Model file for the job. Use its own axes, mm. Face numbers are marked on the shaded views. A direction names the side the tool comes from. Give positions to 0.01 mm unless a question says otherwise; leave off trailing zeros. Loops run counter-clockwise (first coordinate to the right, second up) from the corner with the lowest first, then second, coordinate; pieces in that order, holes last. Notation, with made-up numbers: (-21.75, 14) - (7.25, 14) arc R20 cw to (7.25, 36) - close; hole circle Ø7 at (54.25, -21.75). An arc over 180 degrees is marked (long way). Use a Markdown table: item, result.
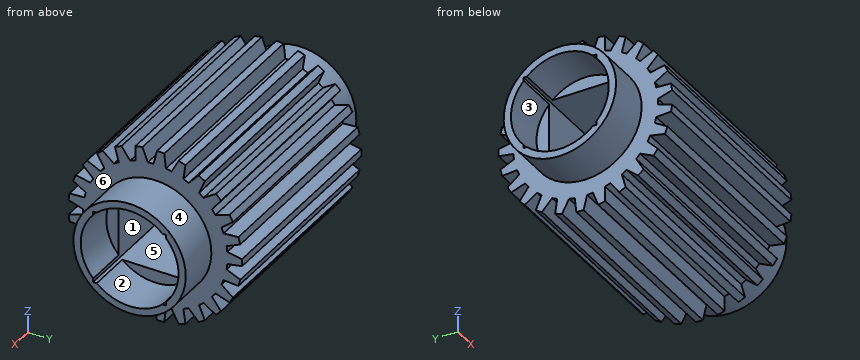
from build123d import *

# Parameters (mm, degrees)
BOSS_EXTRUDE2_START      = -9
BOSS_EXTRUDE2_DEPTH      = 14
BOSS_EXTRUDE3_DEPTH      = 5
BOSS_EXTRUDE3_DEPTH_BACK = 9
SKETCH3_R                = 5
CIRPATTERN1_COUNT        = 25
SKETCH4_W                = 5
SKETCH4_H                = 5
CUT_EXTRUDE1_DEPTH       = 18
BOSS_EXTRUDE4_DEPTH      = 3
BOSS_EXTRUDE4_DEPTH_BACK = 17
SKETCH6_R                = 3.881431072
SKETCH6_R_2              = 3.381431072
CUT_EXTRUDE2_DEPTH       = 10
CUT_EXTRUDE2_DEPTH_BACK  = 20
SKETCH7_W                = 5
SKETCH7_H                = 5.021637953


with BuildPart() as part:
    # Sketch2 → Boss-Extrude2 (new body)
    with BuildSketch(Plane(origin=(0, 0, 0), x_dir=(0, 0, -1), z_dir=(1, 0, 0)).offset(BOSS_EXTRUDE2_START)):
        with BuildLine():
            ThreePointArc((0.429587035, 4.981511315), (0, 5), (-0.429587035, 4.981511315))
            Line((-0.429587035, 4.981511315), (-0.700772987, 3.443539352))
            Line((-0.700772987, 3.443539352), (0.700772987, 3.443539352))
            Line((0.700772987, 3.443539352), (0.429587035, 4.981511315))
        make_face()
        with BuildLine():
            Line((0.25, 6), (-0.25, 6))
            Line((-0.25, 6), (-0.429587035, 4.981511315))
            ThreePointArc((-0.429587035, 4.981511315), (0, 5), (0.429587035, 4.981511315))
            Line((0.429587035, 4.981511315), (0.25, 6))
        make_face()
    boss_extrude2 = extrude(amount=BOSS_EXTRUDE2_DEPTH)

    # Sketch3 → Boss-Extrude3 (add, two sides: drawn at the far end of the back side and taken through both)
    with BuildSketch(Plane(origin=(0, 0, 0), x_dir=(0, 0, -1), z_dir=(1, 0, 0)).offset(-BOSS_EXTRUDE3_DEPTH_BACK)):
        Circle(SKETCH3_R)
    extrude(amount=BOSS_EXTRUDE3_DEPTH + BOSS_EXTRUDE3_DEPTH_BACK)

    # CirPattern1: Boss-Extrude2 ×25 about axis
    cirpattern1_axis = Axis((0, 0, 0), (1, 0, 0))
    for i in range(1, CIRPATTERN1_COUNT):
        add(boss_extrude2.rotate(cirpattern1_axis, i * 360 / CIRPATTERN1_COUNT))

    # Sketch4 → Cut-Extrude1 (cut)
    with BuildSketch(Plane(origin=(5, 0, 0), x_dir=(0, 0, -1), z_dir=(1, 0, 0))):
        Rectangle(SKETCH4_W, SKETCH4_H)
    extrude(amount=-CUT_EXTRUDE1_DEPTH, mode=Mode.SUBTRACT)

    # Sketch6 → Boss-Extrude4 (add, two sides: drawn at the far end of the back side and taken through both)
    with BuildSketch(Plane(origin=(5, 0, 0), x_dir=(0, 0, -1), z_dir=(1, 0, 0)).offset(-BOSS_EXTRUDE4_DEPTH_BACK)):
        Circle(SKETCH6_R)
        Circle(SKETCH6_R_2, mode=Mode.SUBTRACT)
    extrude(amount=BOSS_EXTRUDE4_DEPTH + BOSS_EXTRUDE4_DEPTH_BACK)

    # Sketch7 → Cut-Extrude2 (cut, two sides: drawn at the far end of the back side and taken through both)
    with BuildSketch(Plane(origin=(5, 0, 0), x_dir=(0, 0, -1), z_dir=(1, 0, 0)).offset(-CUT_EXTRUDE2_DEPTH_BACK)):
        with Locations((0, -0.010818977)):
            Rectangle(SKETCH7_W, SKETCH7_H)
    extrude(amount=CUT_EXTRUDE2_DEPTH + CUT_EXTRUDE2_DEPTH_BACK, mode=Mode.SUBTRACT)


solid = part.part
(1) 3-axis set-ups, long thin cutter, end or side, ignore diameter. For the marked faces 1, 2 and 3: which of +Z, -Z, +X, -X, +Y, -Y reach the whole face in a straight line?
Computed:
| item | result |
|---|---|
| face 1 | +X, -X |
| face 2 | +X |
| face 3 | -X |
(2) Slice it at A-A, the plane x = -9.5. Write the cut outline in (y, z), plus the area to 3 significant figures.
Computed:
| item | result |
|---|---|
| outline | circle Ø7.76 at (0, 0); hole (-2.52, -2.5) - (-2.28, -2.5) arc R3.38 ccw to (2.28, -2.5) - (2.5, -2.5) - (2.5, -2.28) arc R3.38 ccw to (2.5, 2.28) - (2.5, 2.5) - (2.28, 2.5) arc R3.38 ccw to (-2.28, 2.5) - (-2.52, 2.5) - (-2.52, 2.25) arc R3.38 ccw to (-2.52, -2.25) - close |
| area | 11.3 mm² |
(3) Pin check, flat tips, straight feed: P1, Ø1, axis at x = -5.5, y = -3.5, coming from the +Z side; P2, Ø0.7, axis at y = 3, z = 0, coming from the -X side; P3, Ø0.7, axis at y = 2.5, z = 0, coming from the +X side. Stop position of each tip, or through.
Computed:
| item | result |
|---|---|
| P1 | z = 4.78 |
| P2 | x = -9 |
| P3 | x = 5 |
(4) Drill centre lines: probe 1 along Z at (x, y) = (-2.75, 4); probe 2 along Z at (x, y) = (0.75, -4.75); probe 3 along Z at (x, y) = (6.5, 0). Where is each one in solid material? Low to high. Write a range as [from, to].
Computed:
| item | result |
|---|---|
| probe 1 | [-4.16, -3.2], [-3, 3], [3.2, 4.16] |
| probe 2 | [-3.67, -3.06], [-2.29, 2.29], [3.06, 3.67] |
| probe 3 | [-3.88, -3.38], [3.38, 3.88] |
(5) Mould opens along Z. For the marked faces 4, 5 and 6 say: pulls with the +Z half, pulls with the -Z half, needs draft (parallel to the pull), parting line crosses it, or undercut.
Computed:
| item | result |
|---|---|
| face 4 | parting line crosses it |
| face 5 | undercut |
| face 6 | needs draft |
